Source: CAD feature listing. Evaluate the final solid. Frame: model axes, mm. Face numbers are marked on the shaded views. A direction names the side the tool comes from. Give positions to 0.01 mm unless a question says otherwise; leave off trailing zeros. Order: outer loops, then holes, each group sorted by start corner. A loop starts at its lowest first (then second) coordinate and runs counter-clockwise, first axis right, second up. Notation, with made-up numbers: M 54,30.5 L 64,30.5 A24 ccw 64,41.5 Z; hole C 17.5,19 d3. An arc over 180 degrees is marked long. Answer as a JSON object with one key per item and string values. Group by question number.
1. Pull-direction query (X, two-part tool) for the marked faces 3, 4 and 5; classes: +X half, -X half, draft (parallel to the pull), parting line (faces both ways), or undercut.
2. Set-up query: the marked faces 1 and 2. Return all of +Z, -Z, +X, -X, +Y, -Y with unobstructed straight access to the full face (end or side cutting, diameter ignored); none if empty.
3. Section query B-B (x = 67). Output: boundary loops of the cut face in (y, z).
4. Material intervals for L1, parallel to Y at x = 35.5, z = 4; L2, parallel to Z at x = -81.5, y = -34.5; L3, parallel to Y at x = 42, z = 6, sorted ascending. Write a range as [from, to].
5. Section query C-C (z = 4.5). Output: boundary loops of the cut face in (x, y).
6. Section query D-D (x = -51.5). Output: boundary loops of the cut face in (y, z), plus the area to 3 significant figures.
7. Section query A-A (y = 40). Output: boundary loops of the cut face in (x, z), plus the area to 3 significant figures.
8. Pin query (flat end, axial travel): P1, Ø8, axis at y = -38.5, z = 31.5, coming from the +X side; P2, Ø12.5, axis at x = -30, z = 26, coming from the -Y side; P3, Ø4, axis at x = -74.5, z = 3.5, coming from the -Y side. Return the tip coordinate at first contact, or that it passes through.
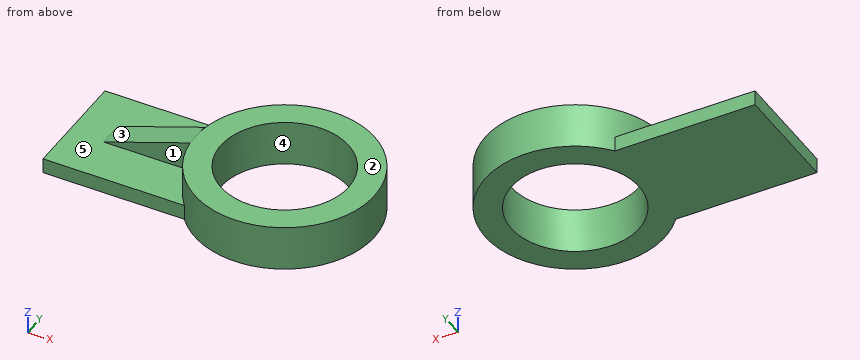
from build123d import *

# Parameters (mm, degrees)
F0_W      = 158.8544994593
F0_H      = 94.7234593332
F1_DEPTH  = 12.7
F3_DEPTH  = 12.701
F4_R      = 75.1836031241
F5_DEPTH  = 38.1
F6_R      = 53.5400409411
F7_DEPTH  = 38.101
F8_W      = 72.6389752571
F8_H      = 21.686675027
F9_DEPTH  = 25.4
F11_DEPTH = 83.5967873179


with BuildPart() as f1:
    # F0 (on Top) → F1 (new body)
    with BuildSketch(Plane.XY):
        with Locations((-31.5255522728, 7.8500341624)):
            Rectangle(F0_W, F0_H)
    extrude(amount=F1_DEPTH)

    # F2 (on face) → F3 (cut, through all)
    with BuildSketch(Plane.XY.offset(12.7)):
        with BuildLine():
            Line((47.9016974568, -39.5116955042), (47.9016974568, 55.211763829))
            ThreePointArc((47.9016974568, 55.211763829), (16.204565289, 7.8500341624), (47.9016974568, -39.5116955042))
        make_face()
    extrude(amount=-F3_DEPTH, mode=Mode.SUBTRACT)

    # F4 (on Top) → F5 (join)
    with BuildSketch(Plane.XY):
        with Locations((65.4443874955, 8.4121841937)):
            Circle(F4_R)
    extrude(amount=F5_DEPTH)

    # F6 (on face) → F7 (cut, through all)
    with BuildSketch(Plane.XY.offset(38.1)):
        with Locations((65.4443874955, 8.4121841937)):
            Circle(F6_R)
    extrude(amount=-F7_DEPTH, mode=Mode.SUBTRACT)

    # F8 (on face) → F9 (join)
    with BuildSketch(Plane.XY.offset(12.7)):
        with Locations((-45.5866075186, 10.8433375135)):
            Rectangle(F8_W, F8_H)
    extrude(amount=F9_DEPTH)

    # F10 (on face) → F11 (cut, through all)
    with BuildSketch(Plane.XZ):
        Polygon((-81.9060951471, 38.1), (-81.9060951471, 12.7), (-9.26711989, 38.1), align=None)
    extrude(amount=-F11_DEPTH, mode=Mode.SUBTRACT)


solid = f1.part
Answer sheet:
{
 "1": {"face 3": "-X half", "face 4": "undercut", "face 5": "draft"},
 "2": {"face 1": "+Z, -X, -Y", "face 2": "+Z, +X, -X, +Y, -Y"},
 "3": {"outline": "M -66.76,0 L -45.11,0 L -45.11,38.1 L -66.76,38.1 Z; M 61.93,0 L 83.58,0 L 83.58,38.1 L 61.93,38.1 Z"},
 "4": {"L1": "[-60.55, -35.97], [52.8, 77.38]", "L2": "[0, 12.7]", "L3": "[-63.02, -39.72], [56.55, 79.85]"},
 "5": {"outline": "M -110.95,-39.51 L 7.51,-39.51 A75.18 ccw long 6.6,55.21 L -110.95,55.21 Z; hole C 65.44,8.41 d107.08"},
 "6": {"outline": "M -39.51,0 L 55.21,0 L 55.21,12.7 L 21.69,12.7 L 21.69,23.33 L 0,23.33 L 0,12.7 L -39.51,12.7 Z", "area": "1,430 mm^2"},
 "7": {"outline": "M -110.95,0 L 22.22,0 L 22.22,38.1 L -2.78,38.1 L -2.78,12.7 L -110.95,12.7 Z; M 108.67,0 L 133.67,0 L 133.67,38.1 L 108.67,38.1 Z", "area": "3,280 mm^2"},
 "8": {"P1": "x = 127.18", "P2": "y = 0", "P3": "y = -39.51"}
}
